Source: CAD feature listing. Evaluate the final solid. Frame: model axes, mm. Face numbers are marked on the shaded views. Round coordinates to 2 decimals unless told otherwise and drop trailing zeros. Order: outer loops, then holes, each group sorted by start corner. A loop starts at its lowest first (then second) coordinate and runs counter-clockwise, first axis right, second up. Notation, with made-up numbers: M -35.75,-39 L -1.75,-39 A24 ccw -1.75,-2 Z; hole C 4.5,-26 d5. An arc over 180 degrees is marked long. Use one line per item in the form item = value. Start each with the question number.
Q1. Section A-A (x = -33). Return the cut outline in (y, z).
Q2. Section B-B (z = 52.5). Return the cut outline in (x, y), plus the area to 3 significant figures.
Q3. Material intervals for probe 1 along Z at (x, y) = (-30, -15.5); probe 2 along Z at (x, y) = (-12, 34.5); probe 3 along X at (y, z) = (17.5, 105), sorted ascending.
Q4. Section C-C (y = -48). Return the cut outline in (x, z).
Q5. Contact query for a flat-ended pin moving along its axis: pin 1 (5.5 mm diameter, centred on y = -3.18, z = 63.85, fed in from -X). Output: stop coordinate, or through.
Q6. Pull-direction query (Y, two-part tool) for the marked faces 1, 2 and 3; classes: pulls with the +Y half, pulls with the -Y half, needs draft (parallel to the pull), parting line crosses it, or undercut.
Q7. Section D-D (y = -2). Return the cut outline in (x, z), plus the area to 3 significant figures.
from build123d import *

# Parameters (mm, degrees)
ESBO_O1_W                = 120
ESBO_O1_H                = 120
RESSALTO_EXTRUS_O1_DEPTH = 120
ESBO_O2_W                = 55
ESBO_O2_H                = 88
CORTE_EXTRUS_O2_DEPTH    = 5
ESBO_O3_W                = 110.936399694
ESBO_O3_H                = 3.5
CORTE_EXTRUS_O3_DEPTH    = 142
ESBO_O4_W                = 7
ESBO_O4_H                = 5
CORTE_EXTRUS_O5_DEPTH    = 2
ESBO_O5_W                = 5
ESBO_O5_H                = 12
CORTE_EXTRUS_O6_DEPTH    = 10
ESBO_O6_R                = 3.961568313
CORTE_EXTRUS_O7_DEPTH    = 230
ESBO_O7_R                = 3.592178765
CORTE_EXTRUS_O8_DEPTH    = 90


with BuildPart() as part:
    # Esboço1 → Ressalto-extrusão1 (new body)
    with BuildSketch(Plane.XY):
        with Locations((-12.702949292, -5.410650407)):
            Rectangle(ESBO_O1_W, ESBO_O1_H)
    extrude(amount=RESSALTO_EXTRUS_O1_DEPTH)

    # Esboço2 → Corte-extrusão2 (cut)
    with BuildSketch(Plane.ZY.offset(72.702949292)):
        with Locations((61.153940809, -6.205937977)):
            Rectangle(ESBO_O2_W, ESBO_O2_H)
    extrude(amount=-CORTE_EXTRUS_O2_DEPTH, mode=Mode.SUBTRACT)

    # Esboço3 → Corte-extrusão3 (cut)
    with BuildSketch(Plane(origin=(0, 54.589349593, 0), x_dir=(1, 0, 0), z_dir=(0, 1, 0))):
        with Locations((-13.409376007, -110.441569905)):
            Rectangle(ESBO_O3_W, ESBO_O3_H)
        with Locations((-13.409376007, -106.084018742)):
            Rectangle(ESBO_O3_W, ESBO_O3_H)
    extrude(amount=-CORTE_EXTRUS_O3_DEPTH, mode=Mode.SUBTRACT)

    # Esboço4 → Corte-extrusão5 (cut)
    with BuildSketch(Plane(origin=(0, 54.589349593, 0), x_dir=(1, 0, 0), z_dir=(0, 1, 0))):
        with Locations((-58.31528793, -10.660946626)):
            Rectangle(ESBO_O4_W, ESBO_O4_H)
    extrude(amount=-CORTE_EXTRUS_O5_DEPTH, mode=Mode.SUBTRACT)

    # Esboço5 → Corte-extrusão6 (cut)
    with BuildSketch(Plane.ZY.offset(72.702949292)):
        with Locations((12.892561397, -49.999881636)):
            Rectangle(ESBO_O5_W, ESBO_O5_H)
    extrude(amount=-CORTE_EXTRUS_O6_DEPTH, mode=Mode.SUBTRACT)

    # Esboço6 → Corte-extrusão7 (cut)
    with BuildSketch(Plane(origin=(0, 54.589349593, 0), x_dir=(1, 0, 0), z_dir=(0, 1, 0))):
        with Locations(Location((-11.856000819, -65.210905781, 0), (0, 0, 270))):
            Circle(ESBO_O6_R)
    extrude(amount=-CORTE_EXTRUS_O7_DEPTH, mode=Mode.SUBTRACT)

    # Esboço7 → Corte-extrusão8 (cut)
    with BuildSketch(Plane(origin=(47.297050708, 0, 0), x_dir=(0, 0, -1), z_dir=(1, 0, 0))):
        with Locations(Location((-63.849475515, -3.180838573, 0), (0, 0, 90))):
            Circle(ESBO_O7_R)
    extrude(amount=-CORTE_EXTRUS_O8_DEPTH, mode=Mode.SUBTRACT)


solid = part.part
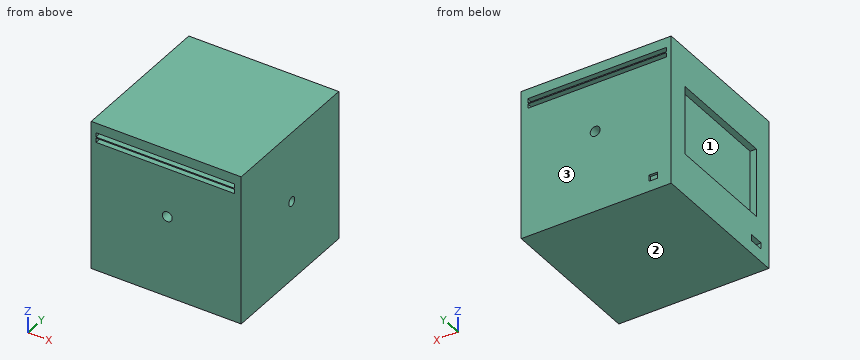
Results list:
q1.outline = M -65.41,0 L 54.59,0 L 54.59,104.33 L -65.41,104.33 Z; M -65.41,107.83 L 54.59,107.83 L 54.59,108.69 L -65.41,108.69 Z; M -65.41,112.19 L 54.59,112.19 L 54.59,120 L -65.41,120 Z; hole C -3.18,63.85 d7.18
q2.outline = M -72.7,-65.41 L 47.3,-65.41 L 47.3,54.59 L -72.7,54.59 L -72.7,37.79 L -67.7,37.79 L -67.7,-50.21 L -72.7,-50.21 Z
q2.area = 14,000 mm2
q3.probe_1 = 0 to 104.33, 107.83 to 108.69, 112.19 to 120
q3.probe_2 = 0 to 61.25, 69.17 to 104.33, 107.83 to 108.69, 112.19 to 120
q3.probe_3 = -72.7 to -68.88, 42.06 to 47.3
q4.outline = M -72.7,0 L 47.3,0 L 47.3,120 L -72.7,120 L -72.7,88.65 L -67.7,88.65 L -67.7,33.65 L -72.7,33.65 L -72.7,15.39 L -62.7,15.39 L -62.7,10.39 L -72.7,10.39 Z; hole M -68.88,104.33 L 42.06,104.33 L 42.06,107.83 L -68.88,107.83 Z; hole M -68.88,108.69 L 42.06,108.69 L 42.06,112.19 L -68.88,112.19 Z; hole C -11.86,65.21 d7.92
q5.pin_1 = -67.7
q6.face_1 = undercut
q6.face_2 = needs draft
q6.face_3 = pulls with the +Y half
q7.outline = M -72.7,0 L 47.3,0 L 47.3,60.46 L -42.7,60.46 L -42.7,67.24 L -15.26,67.24 A3.96 cw -8.45,67.24 L 47.3,67.24 L 47.3,120 L -72.7,120 L -72.7,88.65 L -67.7,88.65 L -67.7,33.65 L -72.7,33.65 Z; hole M -68.88,104.33 L 42.06,104.33 L 42.06,107.83 L -68.88,107.83 Z; hole M -68.88,108.69 L 42.06,108.69 L 42.06,112.19 L -68.88,112.19 Z
q7.area = 12,700 mm2
